Can you work these out from the model? Positions are in its coordinate system, mm. A direction names the side the tool comes from. Coordinates: 2 decimals unless noted, no trailing zeros. Loops run counter-clockwise (first coordinate to the right, second up) from the corner with the lowest first, then second, coordinate; pieces in that order, holes last.
```python
from build123d import *

# Parameters (mm, degrees)
F0_W     = 100
F0_H     = 50
F1_DEPTH = 60
F3_DEPTH = 50.001
F4_W     = 100
F4_H     = 32
F5_DEPTH = 15
F6_W     = 70
F6_H     = 15
F7_DEPTH = 60.001


with BuildPart() as f1:
    # F0 (on Top) → F1 (new body)
    with BuildSketch(Plane.XY):
        with Locations((50, 25)):
            Rectangle(F0_W, F0_H)
    extrude(amount=F1_DEPTH)

    # F2 (on face) → F3 (cut, through all)
    with BuildSketch(Plane.XZ):
        Polygon((15, 60), (0, 60), (0, 40), align=None)
        Polygon((55, 60), (100, 20), (100, 60), align=None)
    extrude(amount=-F3_DEPTH, mode=Mode.SUBTRACT)

    # F4 (on face) → F5 (cut)
    with BuildSketch(Plane.XZ):
        with Locations((50, 16)):
            Rectangle(F4_W, F4_H)
    extrude(amount=-F5_DEPTH, mode=Mode.SUBTRACT)

    # F6 (on face) → F7 (cut, through all)
    with BuildSketch(Plane(origin=(0, 0, 0), x_dir=(1, 0, 0), z_dir=(0, 0, -1))):
        with Locations((65, -42.5)):
            Rectangle(F6_W, F6_H)
    extrude(amount=-F7_DEPTH, mode=Mode.SUBTRACT)


solid = f1.part
```
(1) Which directions (+Z, -Z, +X, -X, +Y, -Y) give clear straight access to the entire face, cutting with the end or side of a thin tool? Please do faces 1 (the flat face through (0, 30, 20)), 2 (the flat face through (43, 7, 32)), 3 (the flat face through (30, 43, 30)).
Check values:
face 1: +Z, -Z, -X, +Y, -Y
face 2: -Z, +X, -X, -Y
face 3: +Z, -Z, +X, +Y
(2) I want a section at B-B on z = 14.5. Write out the boundary of the cut face in (x, y), then the cut area to 3 significant figures.
Check values:
outline: (0, 15) - (100, 15) - (100, 35) - (30, 35) - (30, 50) - (0, 50) - close
area: 2,450 mm2
(3) I want a section at D-D on y = 5.5. Write out the boundary of the cut face in (x, z).
Check values:
outline: (0, 32) - (86.5, 32) - (55, 60) - (15, 60) - (0, 40) - close
(4) I want a section at A-A on y = 43.5. Write out the boundary of the cut face in (x, z).
Check values:
outline: (0, 0) - (30, 0) - (30, 60) - (15, 60) - (0, 40) - close
(5) I want a section at C-C on x = 46. Write out the boundary of the cut face in (y, z), then the cut area to 3 significant figures.
Check values:
outline: (0, 32) - (15, 32) - (15, 0) - (35, 0) - (35, 60) - (0, 60) - close
area: 1,620 mm2
(6) If I drill on probe 1 along X at (y, z) = (39.5, 16.5); probe 2 along Y at (x, z) = (59.5, 8); probe 3 along Y at (x, z) = (18, 10), over which ranges is the centre line in solid material (lowest first)?
Check values:
probe 1: x = 0 to 30
probe 2: y = 15 to 35
probe 3: y = 15 to 50
(7) I'm going to push flat-ended pins straight in: pin 1 (1 mm diameter, centred on x = 19, y = 13, fed in from -Z); pin 2 (10 mm diameter, centred on x = 14.5, y = 27, fed in from +Z); pin 3 (9.5 mm diameter, centred on x = 51, z = 15, fed in from -Y); pin 4 (12 mm diameter, centred on y = 19, z = 48.5, fed in from -X) (3 decimals). Where does each tip first touch, or does it pass through?
Check values:
pin 1: stops at z = 32
pin 2: stops at z = 60
pin 3: stops at y = 15
pin 4: stops at x = 1.875
